from build123d import *

# Parameters (mm, degrees)
SKETCH1_W           = 36
SKETCH1_H           = 16
BOSS_EXTRUDE1_DEPTH = 6
SKETCH2_R           = 1.6
CUT_EXTRUDE1_DEPTH  = 6
CHAMFER1_SIZE       = 7
SKETCH4_R           = 1.6
CUT_EXTRUDE2_DEPTH  = 6
SKETCH5_W           = 7.5
SKETCH5_H           = 4
CUT_EXTRUDE3_DEPTH  = 6
CHAMFER2_SIZE       = 2
SKETCH6_W           = 1.6
SKETCH6_H           = 4
SKETCH6_W_2         = 1.5
CUT_EXTRUDE4_DEPTH  = 3
SKETCH7_W           = 4
SKETCH7_H           = 1.5
CUT_EXTRUDE6_DEPTH  = 7.5
FILLET1_R           = 3
FILLET2_R           = 3
SKETCH8_W           = 4
SKETCH8_H           = 1.5
CUT_EXTRUDE7_DEPTH  = 7.5
FILLET3_R           = 3
SKETCH10_W          = 5.7
SKETCH10_H          = 6.5
CUT_EXTRUDE8_DEPTH  = 2.6
FILLET4_R           = 4.5


# Some blends are built 0.0001 mm under size
with BuildPart() as part:
    # Sketch1 → Boss-Extrude1 (new body)
    with BuildSketch(Plane.XY):
        with Locations((339.581598667, 83.950008978)):
            Rectangle(SKETCH1_W, SKETCH1_H)
    extrude(amount=BOSS_EXTRUDE1_DEPTH)

    # Sketch2 → Cut-Extrude1 (cut)
    with BuildSketch(Plane.XY.offset(6)):
        with Locations((333.581598667, 87.950008978)):
            Circle(SKETCH2_R)
        with Locations((345.581598667, 87.950008978)):
            Circle(SKETCH2_R)
        with Locations((339.581598667, 79.950008978)):
            Circle(SKETCH2_R)
    extrude(amount=-CUT_EXTRUDE1_DEPTH, mode=Mode.SUBTRACT)

    # Chamfer1
    chamfer1_edges = [part.edges().sort_by_distance(p)[0] for p in [
        (357.581598667, 75.950008978, 3),
        (321.581598667, 75.950008978, 3),
    ]]
    chamfer(chamfer1_edges, length=CHAMFER1_SIZE)

    # Sketch4 → Cut-Extrude2 (cut)
    with BuildSketch(Plane.XY.offset(6)):
        with Locations((324.581598667, 87.950008978)):
            Circle(SKETCH4_R)
        with Locations((354.581598667, 87.950008978)):
            Circle(SKETCH4_R)
    extrude(amount=-CUT_EXTRUDE2_DEPTH, mode=Mode.SUBTRACT)

    # Sketch5 → Cut-Extrude3 (cut)
    with BuildSketch(Plane.XY.offset(6)):
        with Locations((325.331598667, 89.950008978)):
            Rectangle(SKETCH5_W, SKETCH5_H)
        with Locations((353.831598667, 89.950008978)):
            Rectangle(SKETCH5_W, SKETCH5_H)
    extrude(amount=-CUT_EXTRUDE3_DEPTH, mode=Mode.SUBTRACT)

    # Chamfer2
    chamfer2_edges = [part.edges().sort_by_distance(p)[0] for p in [
        (329.081598667, 91.950008978, 3),
        (350.081598667, 91.950008978, 3),
    ]]
    chamfer(chamfer2_edges, length=CHAMFER2_SIZE)

    # Sketch6 → Cut-Extrude4 (cut)
    with BuildSketch(Plane(origin=(0, 87.950008978, 0), x_dir=(1, 0, 0), z_dir=(0, 1, 0))):
        with Locations((328.281598667, -3)):
            Rectangle(SKETCH6_W, SKETCH6_H)
        with Locations((350.831598667, -3)):
            Rectangle(SKETCH6_W_2, SKETCH6_H)
    extrude(amount=-CUT_EXTRUDE4_DEPTH, mode=Mode.SUBTRACT)

    # Sketch7 → Cut-Extrude6 (cut)
    with BuildSketch(Plane(origin=(357.581598667, 0, 0), x_dir=(0, 0, -1), z_dir=(1, 0, 0))):
        with Locations((-3, 84.200008978)):
            Rectangle(SKETCH7_W, SKETCH7_H)
    extrude(amount=-CUT_EXTRUDE6_DEPTH, mode=Mode.SUBTRACT)

    # Fillet1
    fillet1_edges = [part.edges().sort_by_distance(p)[0] for p in [
        (351.581598667, 84.950008978, 3),
    ]]
    fillet(fillet1_edges, radius=FILLET1_R - 0.0001)  # a hair under: the kernel refuses the full size

    # Fillet2
    fillet2_edges = [part.edges().sort_by_distance(p)[0] for p in [
        (357.581598667, 84.950008978, 3),
    ]]
    fillet(fillet2_edges, radius=FILLET2_R - 0.0001)  # a hair under: the kernel refuses the full size

    # Sketch8 → Cut-Extrude7 (cut)
    with BuildSketch(Plane.ZY.offset(-321.581598667)):
        with Locations((3, 84.200008978)):
            Rectangle(SKETCH8_W, SKETCH8_H)
    extrude(amount=-CUT_EXTRUDE7_DEPTH, mode=Mode.SUBTRACT)

    # Fillet3
    # the kernel refuses this fillet: 3 mm, written as the material it takes off along each edge
    with BuildSketch(Plane(origin=(327.481598667, 84.950008978, 1), x_dir=(0, 1, 0), z_dir=(0, 0, 1)), Plane(origin=(321.581598667, 84.950008978, 5), x_dir=(0, 1, 0), z_dir=(0, 0, -1))) as fillet3_piece_1:
        with BuildLine():
            CenterArc((FILLET3_R, FILLET3_R), FILLET3_R, 180, 90)
            Line((0, FILLET3_R), (0, 0))
            Line((0, 0), (FILLET3_R, 0))
        make_face()
    extrude(amount=4, mode=Mode.SUBTRACT)

    # Sketch10 → Cut-Extrude8 (cut)
    with BuildSketch(Plane.XY.offset(6)):
        with Locations((333.581598667, 87.950008978)):
            Rectangle(SKETCH10_W, SKETCH10_H)
        with Locations((345.581598667, 87.950008978)):
            Rectangle(SKETCH10_W, SKETCH10_H)
        with Locations((339.581598667, 79.950008978)):
            Rectangle(SKETCH10_W, SKETCH10_H)
    extrude(amount=-CUT_EXTRUDE8_DEPTH, mode=Mode.SUBTRACT)

    # Fillet4
    fillet4_edges = [part.edges().sort_by_distance(p)[0] for p in [
        (350.081598667, 83.450008978, 3),
        (329.081598667, 83.450008978, 3),
    ]]
    fillet(fillet4_edges, radius=FILLET4_R)


solid = part.part
Here's how the part is built. I have some questions about the finished solid (model axes, mm). A direction names the side the tool comes from. Coordinates: 2 decimals unless noted, no trailing zeros. Loops run counter-clockwise (first coordinate to the right, second up) from the corner with the lowest first, then second, coordinate; pieces in that order, holes last. Notation, with made-up numbers: (-40, 60) -> (5, 60) arc R8 ccw to (5, 67) -> close; hole circle Ø7 at (-39.5, 17). An arc over 180 degrees is marked (long way). Use one line per item in the form item = value. Start each with the question number.
(1) Will these pins go through, and if not, where does the flat tip stop? pin 1 (2.5 mm diameter, centred on x = 339.58, y = 79.95, fed in from +Z); pin 2 (3.5 mm diameter, centred on x = 345.58, y = 87.95, fed in from +Z); pin 3 (1.3 mm diameter, centred on y = 81, z = 5, fed in from +X); pin 4 (1.6 mm diameter, centred on y = 89, z = 3.5, fed in from -X).
(2) If we section it at C-C (y = 89): Please give me the cut outline in (x, z), then the cut area to 3 significant figures.
(3) If we section it at D-D (x = 352.5): Please give me the cut outline in (y, z).
(4) If we section it at A-A (z = 1.5): Give the number of separate pieces and of enclosed holes in the cut face, then the cut area to 3 significant figures.
(5) If we section it at B-B (x = 337.5): Please give me the cut outline in (y, z).
(6) On a 3-axis mill with a long thin cutter (end or side, diameter ignored), from which of +Z, -Z, +X, -X, +Y, -Y can I reach the whole of each face in a straight line? I mean faces 1 (the face through (326.598, 85.823, 2.972)), 2 (the face through (339, 84, 6)), 3 (the face through (321.582, 83.2, 2.3)), 4 (the face through (347, 89, 3.4)), 5 (the face through (327, 87.95, 3)). Say none if no direction works.
(7) Please list where these lines run through material, in increasing order: line 1 along X through (y, z) = (89, 4.75); line 2 along X through (y, z) = (88, 3); line 3 along Y through (x, z) = (340, 3.5).
(8) We'd pull the mould along Y, two halves only. Please class faces 6 (the face through (329.082, 89, 3)), 7 (the face through (339, 75.95, 3)), 8 (the face through (343.983, 88.02, 1.724)): pulls with the +Y half, pulls with the -Y half, needs draft (parallel to the pull), parting line crosses it, or undercut.
Verdict:
q1.pin_1 = through
q1.pin_2 = 3.4
q1.pin_3 = 356.28
q1.pin_4 = 329.08
q2.outline = (329.08, 0) -> (332.37, 0) -> (332.37, 3.4) -> (330.73, 3.4) -> (330.73, 6) -> (329.08, 6) -> close; (334.79, 0) -> (344.37, 0) -> (344.37, 3.4) -> (342.73, 3.4) -> (342.73, 6) -> (336.43, 6) -> (336.43, 3.4) -> (334.79, 3.4) -> close; (346.79, 0) -> (350.08, 0) -> (350.08, 6) -> (348.43, 6) -> (348.43, 3.4) -> (346.79, 3.4) -> close
q2.area = 79.9 mm²
q3.outline = (77.87, 0) -> (87.95, 0) -> (87.95, 6) -> (77.87, 6) -> close; hole (83.96, 1) -> (85.79, 1) -> (85.79, 5) -> (83.96, 5) -> close
q4.separate_pieces = 3
q4.enclosed_holes = 3
q4.area = 400 mm²
q5.outline = (75.95, 0) -> (91.95, 0) -> (91.95, 6) -> (83.2, 6) -> (83.2, 3.4) -> (76.7, 3.4) -> (76.7, 6) -> (75.95, 6) -> close
q6.face_1 = none
q6.face_2 = +Z, +X, -X, +Y, -Y
q6.face_3 = +Z, -Z, -X, +Y, -Y
q6.face_4 = +Z
q6.face_5 = +Z, -Z, -X, +Y
q7.line_1 = 329.08 to 330.73, 336.43 to 342.73, 348.43 to 350.08
q7.line_2 = 329.08 to 331.98, 335.18 to 343.98, 347.18 to 350.08
q7.line_3 = 75.95 to 76.7, 83.2 to 91.95
q8.face_6 = needs draft
q8.face_7 = pulls with the -Y half
q8.face_8 = undercut
